For this review, take the finished solid that the model builds, in its own axes (mm). A direction names the side the tool comes from. Give positions to 0.01 mm unless a question says otherwise; leave off trailing zeros. Order: outer loops, then holes, each group sorted by start corner. A loop starts at its lowest first (then second) coordinate and runs counter-clockwise, first axis right, second up. Notation, with made-up numbers: (82, 54.5) - (91, 54.5) arc R25 ccw to (91, 78.5) - close; hole circle Ø11 at (66, 43). An arc over 180 degrees is marked (long way). One line per item, written item: value.
```python
from build123d import *

# Parameters (mm, degrees)
SALIENTE_EXTRUIR1_DEPTH = 25
CORTAR_EXTRUIR1_DEPTH   = 60
CORTAR_EXTRUIR2_DEPTH   = 50
CROQUIS16_R             = 7.5
SALIENTE_EXTRUIR4_DEPTH = 25
CROQUIS19_R             = 7.5
SALIENTE_EXTRUIR5_DEPTH = 25


with BuildPart() as part:
    # Croquis1 → Saliente-Extruir1 (new body)
    with BuildSketch(Plane.XY):
        with BuildLine():
            Line((38.847221771, 29.508698958), (38.847221771, 42.008698958))
            Line((38.847221771, 42.008698958), (-6.152778229, 43.508698958))
            ThreePointArc((-6.152778229, 43.508698958), (-20.152778229, 29.508698958), (-6.152778229, 15.508698958))
            Line((-6.152778229, 15.508698958), (38.847221771, 17.008698958))
            Line((38.847221771, 17.008698958), (38.847221771, 29.508698958))
        make_face()
    extrude(amount=SALIENTE_EXTRUIR1_DEPTH)

    # Croquis5 → Cortar-Extruir1 (cut)
    with BuildSketch(Plane(origin=(0, 0, 0), x_dir=(1, 0, 0), z_dir=(0, 1, 0))):
        with BuildLine():
            Line((25.847221771, 0), (38.847221771, 0))
            Line((38.847221771, 0), (38.847221771, -25))
            Line((38.847221771, -25), (25.847221771, -25))
            ThreePointArc((25.847221771, -25), (38.347221771, -12.5), (25.847221771, 0))
        make_face()
    extrude(amount=CORTAR_EXTRUIR1_DEPTH, mode=Mode.SUBTRACT)

    # Croquis14 → Cortar-Extruir2 (cut)
    with BuildSketch(Plane.XY):
        Polygon((53.899517017, 17.025365624), (35.13924076, 17.025365624), (-30.270251596, 17.025365624), (-30.270251596, 4.764452962), (53.899517017, 4.764452962), align=None)
        Polygon((-30.270251596, 42.025365624), (38.347221771, 42.025365624), (49.932931428, 42.025365624), (49.932931428, 48.139642848), (-30.270251596, 48.139642848), align=None)
    extrude(amount=CORTAR_EXTRUIR2_DEPTH, mode=Mode.SUBTRACT)

    # Croquis16 → Saliente-Extruir4 (add, symmetric)
    with BuildSketch(Plane(origin=(0, 29.508698958, 0), x_dir=(1, 0, 0), z_dir=(0, 1, 0))):
        with Locations(Location((25.847221771, -12.5, 0), (0, 0, 180))):
            Circle(CROQUIS16_R)
    extrude(amount=SALIENTE_EXTRUIR4_DEPTH, both=True)

    # Croquis19 → Saliente-Extruir5 (add, symmetric)
    with BuildSketch(Plane.XY.offset(12.5)):
        with Locations((-6.152778229, 29.508698958)):
            Circle(CROQUIS19_R)
    extrude(amount=SALIENTE_EXTRUIR5_DEPTH, both=True)


solid = part.part
```
(1) Take a section at B-B (y = 24). Write out the cut boundary in (x, z), then the cut area to 3 significant figures.
Answers below:
outline: (-19.02, 0) - (-11.24, 0) - (-11.24, -12.5) - (-1.06, -12.5) - (-1.06, 0) - (25.85, 0) arc R12.5 ccw to (25.85, 25) - (-1.06, 25) - (-1.06, 37.5) - (-11.24, 37.5) - (-11.24, 25) - (-19.02, 25) - close
area: 1,620 mm^2
(2) Take a section at A-A (z = 10). Write out the cut boundary in (x, y).
Answers below:
outline: (-12.49, 17.03) - (18.78, 17.03) - (18.78, 4.51) - (32.92, 4.51) - (32.92, 17.03) - (38.09, 17.03) - (38.09, 42.03) - (32.92, 42.03) - (32.92, 54.51) - (18.78, 54.51) - (18.78, 42.03) - (-12.42, 42.03) arc R14 ccw to start
(3) Machinability: for faces 1 (the face through (27.473, 48.354, 5.178)), 2 (the face through (-11.68, 34.58, -6.16)), 3 (the face through (-11.68, 34.58, 31.34)), 4 (the face through (-6, 30, -12.5)), 5 (the face through (27.473, 10.855, 5.178)), which of the approach directions +Z, -Z, +X, -X, +Y, -Y give a long, thin tool a straight path to every point of the face, cutting with its end or side? Answer none if there is none.
Answers below:
face 1: +Y
face 2: -Z
face 3: +Z
face 4: -Z, +X, -X, +Y, -Y
face 5: -Y
(4) For P1, Ø12.5, axis at x = 13.5, z = 17.5, coming from the +Y side; P2, Ø1.5, axis at x = 2.5, y = 32.5, coming from the -Z side; P3, Ø1.5, axis at x = 28.5, y = 27.5, coming from the -Z side; P4, Ø10, axis at x = 7, z = 17.5, coming from the -Y side, all flat-tipped, find the tip position at first contact; note any pin that passes through.
Answers below:
P1: stops at y = 54.51
P2: stops at z = 0
P3: stops at z = 0.15
P4: stops at y = 17.03
(5) Take a section at C-C (y = 12.5). Write out the cut boundary in (x, z), then the cut area to 3 significant figures.
Answers below:
outline: circle Ø15 at (25.85, 12.5)
area: 177 mm^2
(6) Wall thickness on line 1 (Z direction, x = -13, y = 21.5); line 2 (Y direction, x = -4.5, z = 17); line 3 (X direction, y = 47, z = 16): over which ranges is each line inside the solid? List them lowest first. Write a range as from..to.
Answers below:
line 1: z = 0..25
line 2: y = 17.03..42.03
line 3: x = 19.21..32.48
(7) Take a section at D-D (z = 24). Write out the cut boundary in (x, y), then the cut area to 3 significant figures.
Answers below:
outline: (-12.49, 17.03) - (30.75, 17.03) - (30.75, 42.03) - (-12.42, 42.03) arc R14 ccw to start
area: 1,220 mm^2
